Build history of the part. All positions in model axes, mm. A direction names the side the tool comes from. Coordinates: 2 decimals unless noted, no trailing zeros. Order: outer loops, then holes, each group sorted by start corner. A loop starts at its lowest first (then second) coordinate and runs counter-clockwise, first axis right, second up. Notation, with made-up numbers: (53.5, 1.5) - (67.5, 1.5) arc R23 cw to (67.5, 32.5) - close; hole circle Ø6 at (-34.75, 0). An arc over 180 degrees is marked (long way). One line per item, written item: value.
from build123d import *
from build123d.topology import SkipClean

# Parameters (mm, degrees)
SKETCH1_W           = 22
SKETCH1_H           = 12
BOSS_EXTRUDE1_DEPTH = 16.5
BOSS_EXTRUDE2_DEPTH = 2
SKETCH4_W           = 22
SKETCH4_H           = 12
BOSS_EXTRUDE3_DEPTH = 4
SKETCH5_R           = 5
BOSS_EXTRUDE4_DEPTH = 4
SKETCH7_R           = 3.5
BOSS_EXTRUDE5_DEPTH = 4
BOSS_EXTRUDE6_DEPTH = 1
CUT_EXTRUDE2_REACH  = 40.888


with BuildPart() as part:
    # Sketch1 → Boss-Extrude1 (new body)
    with BuildSketch(Plane(origin=(0, 0, 0), x_dir=(1, 0, 0), z_dir=(0, 1, 0))):
        Rectangle(SKETCH1_W, SKETCH1_H)
    extrude(amount=BOSS_EXTRUDE1_DEPTH)

    # Sketch2 → Boss-Extrude2 (add)
    with BuildSketch(Plane(origin=(0, 16.5, 0), x_dir=(1, 0, 0), z_dir=(0, 1, 0))):
        with BuildLine():
            Line((-15.5, 6), (15.5, 6))
            Line((15.5, 6), (15.5, 0.916515))
            ThreePointArc((15.5, 0.916515), (12.7, 0), (15.5, -0.916515))
            Line((15.5, -0.916515), (15.5, -6))
            Line((15.5, -6), (-15.5, -6))
            Line((-15.5, -6), (-15.5, -0.916515))
            ThreePointArc((-15.5, -0.916515), (-12.7, 0), (-15.5, 0.916515))
            Line((-15.5, 0.916515), (-15.5, 6))
        make_face()
    extrude(amount=BOSS_EXTRUDE2_DEPTH)

    # Sketch4 → Boss-Extrude3 (add)
    with BuildSketch(Plane(origin=(0, 18.5, 0), x_dir=(1, 0, 0), z_dir=(0, 1, 0))):
        Rectangle(SKETCH4_W, SKETCH4_H)
    extrude(amount=BOSS_EXTRUDE3_DEPTH)

    # Sketch5 → Boss-Extrude4 (add)
    with BuildSketch(Plane(origin=(0, 22.5, 0), x_dir=(1, 0, 0), z_dir=(0, 1, 0))):
        with Locations((6, 0)):
            Circle(SKETCH5_R)
    extrude(amount=BOSS_EXTRUDE4_DEPTH)

    # Sketch7 → Boss-Extrude5 (add)
    with BuildSketch(Plane(origin=(0, 26.5, 0), x_dir=(1, 0, 0), z_dir=(0, 1, 0))):
        with Locations(Location((6, 0, 0), (0, 0, 270))):
            Circle(SKETCH7_R)
    extrude(amount=BOSS_EXTRUDE5_DEPTH)

    # Sketch8 → Boss-Extrude6 (add)
    with SkipClean():  # the faces are left unmerged after this step: merging them gives an invalid solid
        with BuildSketch(Plane(origin=(0, 30.5, 0), x_dir=(1, 0, 0), z_dir=(0, 1, 0))):
            with BuildLine():
                Line((5.516407, -3.46643), (-8.710709, -1.481642))
                ThreePointArc((-8.710709, -1.481642), (-9.996409, 0.103599), (-8.504009, 1.495991))
                Line((-8.504009, 1.495991), (5.512894, 3.465938))
                ThreePointArc((5.512894, 3.465938), (6, 3.5), (6.487106, 3.465938))
                Line((6.487106, 3.465938), (20.504009, 1.495991))
                ThreePointArc((20.504009, 1.495991), (21.996409, 0.103599), (20.710709, -1.481642))
                Line((20.710709, -1.481642), (6.483593, -3.46643))
                ThreePointArc((6.483593, -3.46643), (6, -3.5), (5.516407, -3.46643))
            make_face()
        extrude(amount=BOSS_EXTRUDE6_DEPTH)

    # Sketch10 → Cut-Extrude2 (cut, up to next)
    with BuildSketch(Plane(origin=(0, 31.5, 0), x_dir=(1, 0, 0), z_dir=(0, 1, 0)), mode=Mode.PRIVATE) as cut_extrude2_sk1:
        with BuildLine():
            Line((-8.710709, -1.481642), (5.516407, -3.46643))
            ThreePointArc((5.516407, -3.46643), (2.5, -0.001774), (5.512894, 3.465938))
            Line((5.512894, 3.465938), (-8.504009, 1.495991))
            ThreePointArc((-8.504009, 1.495991), (-9.996409, 0.103599), (-8.710709, -1.481642))
        make_face()
    cut_extrude2_tool1 = extrude(cut_extrude2_sk1.sketch, amount=-CUT_EXTRUDE2_REACH, mode=Mode.PRIVATE) & part.part
    add(cut_extrude2_tool1.solids().sort_by_distance((-2.43068, 31.5, 0.003848))[0], mode=Mode.SUBTRACT)


solid = part.part
1. Band-saw the part on A-A, the plane x = -14.25. Give the cut face in (y, z), and give its area (3 significant figures).
Values found:
outline: (16.5, -6) - (18.5, -6) - (18.5, -1.55) - (16.5, -1.55) - close; (16.5, 1.55) - (18.5, 1.55) - (18.5, 6) - (16.5, 6) - close
area: 17.8 mm2
2. 3-axis set-ups, long thin cutter, end or side, ignore diameter. For faces 5 (the face through (11, 8, 0)), 6 (the face through (12, 18.5, 0)), 7 (the face through (-12, 18.5, 0)): which of +Z, -Z, +X, -X, +Y, -Y reach the whole face in a straight line?
Values found:
face 5: +Z, -Z, +X, -Y
face 6: +Z, -Z, +X
face 7: +Z, -Z, -X, +Y
3. Band-saw the part on C-C, the plane y = 2. Give the cut face in (x, z).
Values found:
outline: (-11, -6) - (11, -6) - (11, 6) - (-11, 6) - close
4. Band-saw the part on B-B, the plane x = 6. Give the cut face in (y, z).
Values found:
outline: (0, -6) - (22.5, -6) - (22.5, -5) - (26.5, -5) - (26.5, -3.5) - (31.5, -3.5) - (31.5, 3.5) - (26.5, 3.5) - (26.5, 5) - (22.5, 5) - (22.5, 6) - (0, 6) - close
5. Band-saw the part on D-D, the plane x = 14.25. Give the cut face in (y, z).
Values found:
outline: (16.5, -6) - (18.5, -6) - (18.5, -1.55) - (16.5, -1.55) - close; (16.5, 1.55) - (18.5, 1.55) - (18.5, 6) - (16.5, 6) - close; (30.5, -2.37) - (31.5, -2.37) - (31.5, 2.38) - (30.5, 2.38) - close
6. Probe line 1 along Z through (x, y) = (-14.25, 16.95); line 2 along Y through (x, z) = (9.5, -1.5); line 3 along X through (y, z) = (6, 1.75). List the from-to ranges inside material, lowest first.
Values found:
line 1: z = -6 to -1.55, 1.55 to 6
line 2: y = 0 to 26.5, 30.5 to 31.5
line 3: x = -11 to 11
7. Flat gauge pins, fed straight in: P1, Ø2, axis at y = 20, z = 3.5, coming from the -X side; P2, Ø4, axis at x = -14.25, z = 0, coming from the +Y side; P3, Ø2, axis at x = -13.5, z = 1.5, coming from the -Y side. Where does each tip first touch, or does it go through?
Values found:
P1: stops at x = -11
P2: stops at y = 18.5
P3: stops at y = 16.5
8. Two-plate mould, pull along X, no slides. Class faces 1 (the face through (2, 24, 3)), 2 (the face through (13.7, 30.99, 2.46)), 3 (the face through (12.7, 17.49, -0.05)), 4 (the face through (12, 16.5, 0)): pulls with the +X half, pulls with the -X half, needs draft (parallel to the pull), parting line crosses it, or undercut.
Values found:
face 1: parting line crosses it
face 2: pulls with the +X half
face 3: undercut
face 4: needs draft
